Here's how the part is built. I have some questions about the finished solid (model axes, mm). A direction names the side the tool comes from. Round coordinates to 2 decimals unless told otherwise and drop trailing zeros. Order: outer loops, then holes, each group sorted by start corner. A loop starts at its lowest first (then second) coordinate and runs counter-clockwise, first axis right, second up. Notation, with made-up numbers: M 27.25,20 L 42.25,20 A24 cw 42.25,56 Z; hole C 38,7 d9. An arc over 180 degrees is marked long. Write item = value, one per line. Start each with the question number.
Item 1: I want a section at A-A, the plane x = 4. List the corners of the cut face in (y, z) for me, plus the area to 3 significant figures.
Item 2: For faces 1 (the face through (3.134, 10, 0)), 2 (the face through (-2.667, 3, 0)), 3 (the face through (10.033, 3, 0)), 4 (the face through (9.525, -5, 2)), which set-ups out of +Z, -Z, +X, -X, +Y, -Y let a thin tool reach every point of the face, with its end or its side?
Item 3: I want a section at D-D, the plane y = -12.7. State how many separate pieces and enclosed holes the cut face has, plus the area to 3 significant figures.
Item 4: We'd pull the mould along X, two halves only. Please class faces 5 (the face through (12.04, -4, -2)), 6 (the face through (-12.04, -4, -2)), 7 (the face through (-0.07, -3.174, 0.031)): pulls with the +X half, pulls with the -X half, needs draft (parallel to the pull), parting line crosses it, or undercut.
Item 5: Please list where these lines run through material, in increasing order: L1, parallel to X at y = 4.5, z = 0.1; L2, parallel to X at y = 6, z = 0; L3, parallel to X at y = 10.75, z = 0 (3 decimals).
Item 6: I'm going to push flat-ended pins straight in: P1, Ø1, axis at x = -10.5, z = -0.5, coming from the -Y side; P2, Ø0.6, axis at x = -11.5, z = 0.5, coming from the -Y side; P3, Ø6, axis at x = -1, y = 1.5, coming from the +Z side. Where does each tip first touch, or does it pass through?
Item 7: I want a section at C-C, the plane y = -6. List the corners of the cut face in (x, z) for me (3 decimals), plus the area to 3 significant figures.
Item 8: I want a section at B-B, the plane y = 3.5. List the corners of the cut face in (x, z) for me, plus the area to 3 significant figures.
```python
from build123d import *

# Parameters (mm, degrees)
SKETCH1_W                = 22.609360872
SKETCH1_H                = 4.3815
SKETCH1_W_2              = 7.366
SKETCH1_H_2              = 1.8415
SKETCH1_W_3              = 7.407296779
BOSS_EXTRUDE1_DEPTH      = 6.35
BOSS_EXTRUDE2_REACH      = 15.15
BOSS_EXTRUDE3_START      = 2.19075
BOSS_EXTRUDE3_DEPTH      = 2.19075
SKETCH7_R                = 1.5875
BOSS_EXTRUDE4_DEPTH      = 1.27
MIRROR2_COPY_1_SKETCH_R  = 1.5875
MIRROR2_COPY_1_DEPTH     = 1.27
BOSS_EXTRUDE5_DEPTH      = 6.35
BOSS_EXTRUDE5_DEPTH_BACK = 1.27
SKETCH8_R                = 2.367055436
SKETCH8_R_2              = 1.095375
SKETCH9_W                = 22.609360872
SKETCH9_H                = 6.35
BOSS_EXTRUDE6_DEPTH      = 4.3815
SKETCH10_W               = 6.35
SKETCH10_H               = 1.8415
CUT_EXTRUDE1_DEPTH       = 12.7
SKETCH12_R               = 1.095375
CUT_EXTRUDE2_DEPTH       = 12.7


with BuildPart() as part:
    # Sketch1 → Boss-Extrude1 (new body)
    with BuildSketch(Plane(origin=(0, 0, 0), x_dir=(1, 0, 0), z_dir=(0, 1, 0))):
        Rectangle(SKETCH1_W, SKETCH1_H)
        with Locations((-6.35, 0)):
            Rectangle(SKETCH1_W_2, SKETCH1_H_2, mode=Mode.SUBTRACT)
        with Locations((6.329351611, 0)):
            Rectangle(SKETCH1_W_3, SKETCH1_H_2, mode=Mode.SUBTRACT)
    extrude(amount=BOSS_EXTRUDE1_DEPTH)

    # Boss-Extrude2: up to this face of the body (flat: up to its plane)
    boss_extrude2_end = Plane(part.part.faces().sort_by_distance((0, 3.175, -2.19075))[0])
    # Sketch2 → Boss-Extrude2 (add, up to the picked face)
    with BuildSketch(Plane.XY, mode=Mode.PRIVATE) as boss_extrude2_sk1:
        with BuildLine():
            Line((3.175, 0), (-3.175, 0))
            ThreePointArc((-3.175, 0), (0, -3.175), (3.175, 0))
        make_face()
    boss_extrude2_tool1 = split(extrude(boss_extrude2_sk1.sketch, amount=-BOSS_EXTRUDE2_REACH, mode=Mode.PRIVATE), bisect_by=boss_extrude2_end, keep=Keep.BOTH, mode=Mode.PRIVATE)
    add(boss_extrude2_tool1.solids().sort_by(Axis((0, -1.347512, 0), (0, 0, -1)))[0])

    # Sketch2<3> → Boss-Extrude3 (add)
    with BuildSketch(Plane.XY.offset(BOSS_EXTRUDE3_START)):
        with BuildLine():
            Line((3.175, 0), (-3.175, 0))
            ThreePointArc((-3.175, 0), (0, -3.175), (3.175, 0))
        make_face()
    extrude(amount=-BOSS_EXTRUDE3_DEPTH)

    # Sketch7 → Boss-Extrude4 (add)
    with BuildSketch(Plane.XY.offset(2.19075)):
        with BuildLine():
            Line((-9.525, 0), (-9.525, -10.16))
            ThreePointArc((-9.525, -10.16), (-7.860334077, -14.618459634), (-12.039641241, -12.341978452))
            Line((-12.039641241, -12.341978452), (-12.039641241, 0))
            Line((-12.039641241, 0), (-12.039641241, 6.35))
            Line((-12.039641241, 6.35), (-11.304680436, 6.35))
            Line((-11.304680436, 6.35), (-11.304680436, 0))
            Line((-11.304680436, 0), (-9.525, 0))
        make_face()
        with Locations((-9.525, -12.7)):
            Circle(SKETCH7_R, mode=Mode.SUBTRACT)
    boss_extrude4 = extrude(amount=-BOSS_EXTRUDE4_DEPTH)

    # Mirror1: Boss-Extrude4 across plane
    add(boss_extrude4.mirror(Plane(origin=(0, 0, 0), x_dir=(0, 0, 1), z_dir=(1, 0, 0))))

    # Mirror2: Boss-Extrude4 across plane
    add(boss_extrude4.mirror(Plane.XY))

    # Mirror2 copy 1 sketch → Mirror2 copy 1 (add)
    with BuildSketch(Plane(origin=(0, 0, -2.19075), x_dir=(-1, 0, 0), z_dir=(0, 0, -1))):
        with BuildLine():
            Line((-9.525, 0), (-9.525, -10.16))
            ThreePointArc((-9.525, -10.16), (-7.860334077, -14.618459634), (-12.039641241, -12.341978452))
            Line((-12.039641241, -12.341978452), (-12.039641241, 0))
            Line((-12.039641241, 0), (-12.039641241, 6.35))
            Line((-12.039641241, 6.35), (-11.304680436, 6.35))
            Line((-11.304680436, 6.35), (-11.304680436, 0))
            Line((-11.304680436, 0), (-9.525, 0))
        make_face()
        with Locations((-9.525, -12.7)):
            Circle(MIRROR2_COPY_1_SKETCH_R, mode=Mode.SUBTRACT)
    extrude(amount=-MIRROR2_COPY_1_DEPTH)

    # Sketch8 → Boss-Extrude5 (add, two sides: drawn at the far end of the back side and taken through both)
    # profile 1 of 2: a face of its own
    with BuildSketch(Plane(origin=(0, 6.35, 0), x_dir=(1, 0, 0), z_dir=(0, 1, 0)).offset(-BOSS_EXTRUDE5_DEPTH_BACK)):
        with Locations(Location((-12.400055436, 0, 0), (0, 0, 67.746440803))):
            Circle(SKETCH8_R)
        with Locations(Location((-12.400055436, 0, 0), (0, 0, 70.789925107))):
            Circle(SKETCH8_R_2, mode=Mode.SUBTRACT)
    # profile 2 of 2: a face of its own
    with BuildSketch(Plane(origin=(0, 6.35, 0), x_dir=(1, 0, 0), z_dir=(0, 1, 0)).offset(-BOSS_EXTRUDE5_DEPTH_BACK)):
        with Locations(Location((12.400055436, 0, 0), (0, 0, 90))):
            Circle(SKETCH8_R)
        with Locations(Location((12.400055436, 0, 0), (0, 0, 90))):
            Circle(SKETCH8_R_2, mode=Mode.SUBTRACT)
    extrude(amount=BOSS_EXTRUDE5_DEPTH + BOSS_EXTRUDE5_DEPTH_BACK)

    # Sketch9 → Boss-Extrude6 (add)
    with BuildSketch(Plane(origin=(0, 0, -2.19075), x_dir=(-1, 0, 0), z_dir=(0, 0, -1))):
        with Locations((0, 9.525)):
            Rectangle(SKETCH9_W, SKETCH9_H)
    extrude(amount=-BOSS_EXTRUDE6_DEPTH)

    # Sketch10 → Cut-Extrude1 (cut)
    with BuildSketch(Plane(origin=(0, 12.7, 0), x_dir=(1, 0, 0), z_dir=(0, 1, 0))):
        with Locations((6.308703221, 0)):
            Rectangle(SKETCH10_W, SKETCH10_H)
        with Locations((-6.35, 0)):
            Rectangle(SKETCH10_W, SKETCH10_H)
    extrude(amount=-CUT_EXTRUDE1_DEPTH, mode=Mode.SUBTRACT)

    # Sketch12 → Cut-Extrude2 (cut)
    with BuildSketch(Plane(origin=(0, 12.7, 0), x_dir=(1, 0, 0), z_dir=(0, 1, 0))):
        with Locations(Location((-12.400055436, 0, 0), (0, 0, 70.789925107))):
            Circle(SKETCH12_R)
        with Locations(Location((12.400055436, 0, 0), (0, 0, 90))):
            Circle(SKETCH12_R)
    extrude(amount=-CUT_EXTRUDE2_DEPTH, mode=Mode.SUBTRACT)


solid = part.part
```
Filled in:
q1.outline = M 0,-2.19 L 12.7,-2.19 L 12.7,-0.92 L 0,-0.92 Z; M 0,0.92 L 12.7,0.92 L 12.7,2.19 L 0,2.19 Z
q1.area = 32.3 mm^2
q2.face_1 = +Y
q2.face_2 = none
q2.face_3 = -Y
q2.face_4 = +Z, -Z
q3.separate_pieces = 8
q3.enclosed_holes = 0
q3.area = 9.68 mm^2
q4.face_5 = pulls with the +X half
q4.face_6 = pulls with the -X half
q4.face_7 = undercut
q5.L1 = -11.3 to -10.03, -2.67 to 2.63, 10.03 to 11.3
q5.L2 = -14.77 to -13.5, -11.3 to -10.03, -2.67 to 2.63, 10.03 to 11.3, 13.5 to 14.77
q5.L3 = -14.767 to -13.495, -11.305 to -9.525, -3.175 to 3.134, 9.484 to 11.305, 13.495 to 14.767
q6.P1 = -15.14
q6.P2 = 0
q6.P3 = 2.19
q7.outline = M -12.04,-2.191 L -9.525,-2.191 L -9.525,-0.921 L -12.04,-0.921 Z; M -12.04,0.921 L -9.525,0.921 L -9.525,2.191 L -12.04,2.191 Z; M 9.525,-2.191 L 12.04,-2.191 L 12.04,-0.921 L 9.525,-0.921 Z; M 9.525,0.921 L 12.04,0.921 L 12.04,2.191 L 9.525,2.191 Z
q7.area = 12.8 mm^2
q8.outline = M -12.04,-2.19 L 12.04,-2.19 L 12.04,-1.03 A1.1 cw 11.81,-0.92 L 11.3,-0.92 L 11.3,0.92 L 11.81,0.92 A1.1 cw 12.04,1.03 L 12.04,2.19 L -12.04,2.19 L -12.04,1.03 A1.1 cw -11.81,0.92 L -11.3,0.92 L -11.3,-0.92 L -11.81,-0.92 A1.1 cw -12.04,-1.03 Z; hole M -10.03,-0.92 L -2.67,-0.92 L -2.67,0.92 L -10.03,0.92 Z; hole M 2.63,-0.92 L 10.03,-0.92 L 10.03,0.92 L 2.63,0.92 Z
q8.area = 75.5 mm^2
